Autodesk Inventor part; units mm, degrees
ref_plane "YZ Plane" through (0, 0, 0) normal (1, 0, 0) x (0, 1, 0)
ref_plane "XZ Plane" through (0, 0, 0) normal (0, 1, 0) x (-1, 0, 0)
ref_plane "XY Plane" through (0, 0, 0) normal (0, 0, 1) x (1, 0, 0)
sketch "Sketch1" plane through (0, 0, 0) normal (0, 1, 0) x (-1, 0, 0)
  line L0 (0, 0) -> (25.4, 0)
  line L1 (25.4, 0) -> (25.4, -76.2)
  line L2 (25.4, -76.2) -> (0, -76.2)
  line L3 (0, -76.2) -> (0, 0)
  dimension "d0" = 25.4
  dimension "d1" = 76.2
extrude "Extrusion1" add sketch "Sketch1" along normal blind 6.35
sketch "Sketch2" plane through (0, 6.35, 0) normal (0, 1, 0) x (1, 0, 0)
  line L0 (-25.4, 0) -> (0, 0)
  line L1 (-25.4, 76.2) -> (-25.4, 0)
  line L2 (0, 0) -> (-25.4, 0)
  line L3 (-25.4, 0) -> (-25.4, 4.7625)
  line L4 (-25.4, 4.7625) -> (0, 4.7625)
  line L5 (0, 4.7625) -> (0, 0)
  line L6 (-12.7, 4.7625) -> (-11.43, 4.7625)
  line L7 (-11.43, 4.7625) -> (-13.97, 4.7625)
  line L8 (-13.97, 4.7625) -> (-13.97, 80.9625)
  line L9 (-13.97, 80.9625) -> (-11.43, 80.9625)
  line L10 (-11.43, 80.9625) -> (-11.43, 4.7625)
  line L11 (-13.97, 4.7625) -> (-13.97, 48.4505)
  line L12 (-13.97, 48.4505) -> (0, 48.4505)
  line L13 (0, 0) -> (0, 76.2)
  line L14 (0, 48.4505) -> (-25.4, 48.4505)
  line L15 (-25.4, 48.4505) -> (-25.4, 49.0855)
  line L16 (-25.4, 49.0855) -> (0, 49.0855)
  line L17 (0, 49.0855) -> (0, 48.4505)
  point P0 (-11.43, 48.4505)
  point P1 (0, 49.0855)
  point P2 (-13.97, 49.0855)
  point P3 (-11.43, 49.0855)
  dimension "d4" = 4.7625
  dimension "d5" = 1.27
  dimension "d6" = 2.54
  dimension "d7" = 76.2
  dimension "d8" = 43.688
  dimension "d9" = 25.4
  dimension "d10" = 0.635
extrude "Extrusion2" add sketch "Sketch2" along normal blind 6.35 contours L1 L4 L5 L0
extrude "Extrusion3" cut sketch "Sketch2" against normal blind 1.27 contours L8 L12 L10 L4 | L8 L16 L10 L12 | L8 L9 L10 L16
extrude "Extrusion4" cut sketch "Sketch2" against normal blind 2.54 contours L1 L16 L8 L14 | L12 L10 L16 L13 | L8 L16 L10 L12
properties part number "Capillary Cutting Fixture for O-ring system"
Geometry check sheet. Reference: the model listing, model coordinates, mm. A direction names the side the tool comes from. Give positions to 0.01 mm unless a question says otherwise; leave off trailing zeros. Write each loop counter-clockwise with the first axis right and the second up, starting at its lowest first coordinate (ties: lowest second). Pieces come first, ordered by that corner, then holes. Notation, with made-up numbers: M 34.5,32 L 82.5,32 A22 cw 82.5,52 Z; hole C 63,-23 d4. An arc over 180 degrees is marked long. One line per question, with ' | ' between items.
1. Gauge pin test, flat ends, axial feed: pin 1 (9 mm diameter, centred on x = -18, z = -37.5, fed in from +Y); pin 2 (1.3 mm diameter, centred on x = -13, z = -68, fed in from +Y). Record the tip position at first contact, or that the pin passes through.
Ans:
pin 1: y = 6.35 | pin 2: y = 5.08
2. Set-up check for faces 1 (the face through (-13.97, 6, -62)), 2 (the face through (-13, 6, 0)), 3 (the face through (-6, 6.35, -62)), 4 (the face through (-12.9, 4.8, -49.086)): record each of +Z, -Z, +X, -X, +Y, -Y from which the full face is reachable in a straight line by a thin tool's end or side.
Ans:
face 1: -Z, +Y | face 2: +Z, +X, -X, +Y, -Y | face 3: -Z, +X, -X, +Y | face 4: +X, -X, +Y
3. Cross-section at A-A (x = -23.5). Enter the section's corners in (y, z).
Ans:
outline: M 0,-76.2 L 6.35,-76.2 L 6.35,-49.09 L 3.81,-49.09 L 3.81,-48.45 L 6.35,-48.45 L 6.35,-4.76 L 12.7,-4.76 L 12.7,0 L 0,0 Z
4. Cross-section at D-D (y = 9). Enter the section's corners in (x, z).
Ans:
outline: M -25.4,-4.76 L 0,-4.76 L 0,0 L -25.4,0 Z
5. Cross-section at B-B (z = -43). Enter the section's corners in (x, y).
Ans:
outline: M -25.4,0 L 0,0 L 0,6.35 L -11.43,6.35 L -11.43,5.08 L -13.97,5.08 L -13.97,6.35 L -25.4,6.35 Z
6. Scan lines: line 1 along Z through (x, y) = (-9.25, 5.5); line 2 along X through (y, z) = (5.5, -47.5); line 3 along Z through (x, y) = (-14.75, 7.25). Record each from-to range of solid material in increasing order. Write a range as from..to.
Ans:
line 1: -76.2..-49.09, -48.45..0 | line 2: -25.4..-13.97, -11.43..0 | line 3: -4.76..0
7. Mould release check, pull along Z, two halves, no side actions. Record for faces 5 (the face through (-20, 6.35, -62)), 6 (the face through (-13, 3, -76.2)), 7 (the face through (-12.5, 4.8, -48.45)): released by +Z, released by -Z, zero draft, split by the parting line, or undercut.
Ans:
face 5: zero draft | face 6: released by -Z | face 7: undercut
8. Cross-section at C-C (x = -12.75). Enter the section's corners in (y, z).
Ans:
outline: M 0,-76.2 L 5.08,-76.2 L 5.08,-49.09 L 3.81,-49.09 L 3.81,-48.45 L 5.08,-48.45 L 5.08,-4.76 L 12.7,-4.76 L 12.7,0 L 0,0 Z
